CAD build for the part. Positions are in the model's coordinates, mm. A direction names the side the tool comes from. Coordinates: 2 decimals unless noted, no trailing zeros. Order: outer loops, then holes, each group sorted by start corner. A loop starts at its lowest first (then second) coordinate and runs counter-clockwise, first axis right, second up. Notation, with made-up numbers: M 46,25 L 73,25 A24 cw 73,58 Z; hole C 28.25,24.25 d1. An arc over 180 degrees is marked long. Write item = value, one per line. Start each with the question number.
Autodesk Fusion 360 part; units mm, degrees
sketch "Sketch1" plane through (0, 0, 0) normal (0, 0, 1) x (1, 0, 0)
  line L0 (17, -8) -> (-17, -8)
  line L1 (-17, -8) -> (-17, 8)
  line L2 (-17, 8) -> (17, 8)
  line L3 (17, 8) -> (17, -8)
  line L4 (17, -8) -> (-17, 8) construction
  line L5 (-17, -8) -> (17, 8) construction
  dimension "d1" = 34
  dimension "d2" = 16
extrude "Extrude1" add sketch "Sketch1" along normal blind 16
sketch "Sketch2" plane through (0, 0, 16) normal (0, 0, 1) x (-1, 0, 0)
  line L0 (-17, -8) -> (17, -8)
  line L1 (17, -8) -> (17, 8)
  line L2 (17, 8) -> (-17, 8)
  line L3 (-17, 8) -> (-17, -8)
  line L4 (-17, 8) -> (-15, 8)
  line L5 (-15, 8) -> (-15, -8)
  line L6 (-15, -8) -> (-17, -8)
  line L7 (-17, -8) -> (-17, 8)
  dimension "d5" = 2
extrude "Extrude2" cut sketch "Sketch2" against normal blind 6 contours L0 L2 L3 L4 L5 L6 L7
sketch "Sketch3" plane through (0, 8, 0) normal (0, 1, 0) x (-1, 0, 0)
  line L0 (-15, 16) -> (-15, 10)
  line L1 (-15, 10) -> (-17, 10)
  line L2 (-17, 10) -> (-17, 0)
  line L3 (-17, 0) -> (17, 0)
  line L4 (17, 0) -> (17, 16)
  line L5 (17, 16) -> (-15, 16)
  spline S0 degree 5 poles (-15, 10) (-14.9556, 10.1956) (-14.8603, 10.5802) (-14.6976, 11.1373) (-14.4407, 11.8398) (-14.0484, 12.6464) (-13.5785, 13.3749) (-13.0248, 14.0189) (-12.3836, 14.5751) (-11.6585, 15.0467) (-10.8558, 15.4401) (-10.1566, 15.6975) (-9.6022, 15.8603) (-9.2194, 15.9556) (-9.0247, 16) knots 0 0 0 0 0 0 0.1 0.2 0.3 0.4 0.5 0.6 0.7 0.8 0.9 1 1 1 1 1 1
  point P0 (-13, 14)
extrude "Extrude3" cut sketch "Sketch3" against normal blind 16 contours L0 L5 S0
sketch "Sketch4" plane through (17, 0, 0) normal (1, 0, 0) x (0, 1, 0)
  line L0 (8, 10) -> (-8, 10)
  line L1 (-8, 10) -> (-8, 0)
  line L2 (-8, 0) -> (8, 0)
  line L3 (8, 0) -> (8, 10)
  line L4 (4, 0) -> (-4, 0)
  line L5 (-4, 0) -> (-4, 4)
  line L6 (-4, 4) -> (4, 4)
  line L7 (4, 4) -> (4, 0)
  line L8 (4, 0) -> (-4, 4) construction
  line L9 (-4, 0) -> (4, 4) construction
  point P0 (0, 2)
  dimension "d10" = 8
  dimension "d11" = 4
extrude "Extrude4" cut sketch "Sketch4" against normal blind 34 contours L2 L4 L5 L6 L7
sketch "Sketch5" plane through (17, 0, 0) normal (1, 0, 0) x (0, 1, 0)
  line L0 (4, 4) -> (4, 0)
  line L1 (4, 0) -> (8, 0)
  line L2 (8, 0) -> (8, 10)
  line L3 (8, 10) -> (-8, 10)
  line L4 (-8, 10) -> (-8, 0)
  line L5 (-8, 0) -> (-4, 0)
  line L6 (-4, 0) -> (-4, 4)
  line L7 (-4, 4) -> (4, 4)
  line L8 (2, 4) -> (-2, 4)
  line L9 (-2, 4) -> (-2, 8)
  line L10 (-2, 8) -> (2, 8)
  line L11 (2, 8) -> (2, 4)
  line L12 (2, 4) -> (-2, 8) construction
  line L13 (-2, 4) -> (2, 8) construction
  point P0 (0, 6)
  dimension "d14" = 4
  dimension "d15" = 4
extrude "Extrude5" cut sketch "Sketch5" against normal blind 34 contours L7 L8 L9 L10 L11
sketch "Sketch6" plane through (0, 0, 16) normal (0, 0, 1) x (-1, 0, 0)
  line L0 (-9.0247, 8) -> (-9.0247, -8)
  line L1 (-9.0247, -8) -> (17, -8)
  line L2 (17, -8) -> (17, 8)
  line L3 (17, 8) -> (-9.0247, 8)
  line L4 (-9, -2) -> (11, -2)
  line L5 (11, -2) -> (11, -8)
  line L6 (11, -8) -> (-9, -8)
  line L7 (-9, -8) -> (-9, -2)
  line L8 (-9, -2) -> (11, -8) construction
  line L9 (11, -2) -> (-9, -8) construction
  point P0 (1, -5)
  dimension "d18" = 20
  dimension "d19" = 6
extrude "Extrude6" cut sketch "Sketch6" against normal blind 10 contours L1 L4 L5 L6 L7
sketch "Sketch7" plane through (0, 0, 16) normal (0, 0, 1) x (-1, 0, 0)
  line L0 (-9, -8) -> (-9, -2)
  line L1 (-9, -2) -> (11, -2)
  line L2 (11, -2) -> (11, -8)
  line L3 (11, -8) -> (17, -8)
  line L4 (17, -8) -> (17, 8)
  line L5 (17, 8) -> (-9.0247, 8)
  line L6 (-9.0247, 8) -> (-9.0247, -8)
  line L7 (-9.0247, -8) -> (-9, -8)
  line L8 (11, 2) -> (-9, 2)
  line L9 (-9, 2) -> (-9, 8)
  line L10 (-9, 8) -> (11, 8)
  line L11 (11, 8) -> (11, 2)
  line L12 (11, 2) -> (-9, 8) construction
  line L13 (-9, 2) -> (11, 8) construction
  point P0 (1, 5)
  dimension "d22" = 20
  dimension "d23" = 6
extrude "Extrude7" cut sketch "Sketch7" against normal blind 10 contours L5 L8 L9 L10 L11
sketch "Sketch8" plane through (0, 0, 16) normal (0, 0, 1) x (-1, 0, 0)
  line L0 (11, 8) -> (11, 2)
  line L1 (11, 2) -> (-9, 2)
  line L2 (-9, 2) -> (-9, 8)
  line L3 (-9, 8) -> (-9.0247, 8)
  line L4 (-9.0247, 8) -> (-9.0247, -8)
  line L5 (-9.0247, -8) -> (-9, -8)
  line L6 (-9, -8) -> (-9, -2)
  line L7 (-9, -2) -> (11, -2)
  line L8 (11, -2) -> (11, -8)
  line L9 (11, -8) -> (17, -8)
  line L10 (17, -8) -> (17, 8)
  line L11 (17, 8) -> (11, 8)
  line L12 (11, -2) -> (-9, -2)
  line L13 (-9, -2) -> (-9, 2)
  line L14 (-9, 2) -> (11, 2)
  line L15 (11, 2) -> (11, -2)
  line L16 (11, -2) -> (-9, 2) construction
  line L17 (-9, -2) -> (11, 2) construction
  point P0 (1, 0)
extrude "Extrude8" cut sketch "Sketch8" against normal blind 8 contours L1 L7 L12 L13 L14 L15
sketch "Sketch9" plane through (0, 0, 16) normal (0, 0, 1) x (-1, 0, 0)
  line L0 (11, 8) -> (11, -8)
  line L1 (11, -8) -> (17, -8)
  line L2 (17, -8) -> (17, 8)
  line L3 (17, 8) -> (11, 8)
  line L4 (11, -8) -> (17, -8)
  line L5 (17, -8) -> (17, -4)
  line L6 (17, -4) -> (11, -4)
  line L7 (11, -4) -> (11, -8)
  dimension "d28" = 4
extrude "Extrude9" cut sketch "Sketch9" against normal blind 6 contours L0 L1 L2 L4 L5 L6 L7
sketch "Sketch10" plane through (0, 0, 16) normal (0, 0, 1) x (-1, 0, 0)
  line L0 (11, -4) -> (17, -4)
  line L1 (17, -4) -> (17, 8)
  line L2 (17, 8) -> (11, 8)
  line L3 (11, 8) -> (11, -4)
  line L4 (11, 8) -> (17, 8)
  line L5 (17, 8) -> (17, 4)
  line L6 (17, 4) -> (11, 4)
  line L7 (11, 4) -> (11, 8)
  dimension "d31" = 6
  dimension "d32" = 4
extrude "Extrude10" cut sketch "Sketch10" against normal blind 6 contours L1 L2 L3 L4 L5 L6 L7
sketch "Sketch11" plane through (-11, 0, 0) normal (1, 0, 0) x (0, 1, 0)
  line L0 (-4, 16) -> (-4, 10)
  line L1 (-4, 10) -> (-8, 10)
  line L2 (-8, 10) -> (-8, 6)
  line L3 (-8, 6) -> (-2, 6)
  line L4 (-2, 6) -> (-2, 8)
  line L5 (-2, 8) -> (2, 8)
  line L6 (2, 8) -> (2, 6)
  line L7 (2, 6) -> (8, 6)
  line L8 (8, 6) -> (8, 10)
  line L9 (8, 10) -> (4, 10)
  line L10 (4, 10) -> (4, 16)
  line L11 (4, 16) -> (-4, 16)
sketch "Sketch12" plane through (-17, 0, 0) normal (-1, 0, 0) x (0, -1, 0)
  line L0 (4, 10) -> (4, 16)
  line L1 (4, 16) -> (-4, 16)
  line L2 (-4, 16) -> (-4, 10)
  line L3 (-4, 10) -> (-8, 10)
  line L4 (-8, 10) -> (-8, 0)
  line L5 (-8, 0) -> (-4, 0)
  line L6 (-4, 0) -> (-4, 4)
  line L7 (-4, 4) -> (-2, 4)
  line L8 (-2, 4) -> (-2, 8)
  line L9 (-2, 8) -> (2, 8)
  line L10 (2, 8) -> (2, 4)
  line L11 (2, 4) -> (4, 4)
  line L12 (4, 4) -> (4, 0)
  line L13 (4, 0) -> (8, 0)
  line L14 (8, 0) -> (8, 10)
  line L15 (8, 10) -> (4, 10)
  arc A0 (4, 10) -> (-4, 10) centre (0, 10) ccw
extrude "Extrude11" cut sketch "Sketch12" against normal blind 6 contours L0 L1 L2 A0
1. Mould opens along X. For faces 6 (the flat face through (-11, 0, 9)), 7 (the flat face through (0, -6, 0)), 8 (the flat face through (-17, -0.1, 8.5)) say: released by +X, released by -X, zero draft, split by the parting line, or undercut.
2. Slice it at B-B (z = 4.5). Write the cut outline in (x, y), plus the area to 3 significant figures.
3. 3-axis set-ups, long thin cutter, end or side, ignore diameter. For faces 1 (the flat face through (9, 0, 11)), 2 (the flat face through (0, 4, 2)), 3 (the flat face through (-14, -6, 10)), 4 (the flat face through (16, 0, 10)), 5 (the cylindrical face through (-14, 0, 14)): which of +Z, -Z, +X, -X, +Y, -Y reach the whole face in a straight line?
4. Slice it at A-A (x = 1). Write the cut outline in (y, z), plus the area to 3 significant figures.
5. Flat gauge pins, fed straight in: pin 1 (1 mm diameter, centred on x = 2, y = -3, fed in from -Z); pin 2 (1.8 mm diameter, centred on x = -2.5, y = 4, fed in from +Z); pin 3 (0.6 mm diameter, centred on x = 16.5, y = -1.5, fed in from +Z). Where does each tip first touch, or does it go through?
6. Probe L1, parallel to Y at x = 15, z = 3.75; L2, parallel to X at y = 3, z = 6.75; L3, parallel to Z at x = -14.5, y = -6.25. List the from-to ranges inside material, lowest first.
Calculated:
q1.face_6 = undercut
q1.face_7 = zero draft
q1.face_8 = released by -X
q2.outline = M -17,-8 L 17,-8 L 17,-2 L -17,-2 Z; M -17,2 L 17,2 L 17,8 L -17,8 Z
q2.area = 408 mm²
q3.face_1 = +Z, +Y, -Y
q3.face_2 = -Z, +X, -X
q3.face_3 = +Z, -X, -Y
q3.face_4 = +Z, +X, +Y, -Y
q3.face_5 = +Z, -X
q4.outline = M -8,0 L -4,0 L -4,4 L -2,4 L -2,6 L -8,6 Z; M 2,4 L 4,4 L 4,0 L 8,0 L 8,6 L 2,6 Z
q4.area = 56.0 mm²
q5.pin_1 = 4
q5.pin_2 = 6
q5.pin_3 = 10
q6.L1 = -8 to -4, 4 to 8
q6.L2 = -17 to -11, 9 to 17
q6.L3 = 0 to 10
